Check sheet for the modelled part. Datum: model origin and axes. Units: mm. Face numbers are marked on the shaded views. A direction names the side the tool comes from. Round coordinates to 2 decimals unless told otherwise and drop trailing zeros. Order: outer loops, then holes, each group sorted by start corner. A loop starts at its lowest first (then second) coordinate and runs counter-clockwise, first axis right, second up.
```python
from build123d import *

# Parameters (mm, degrees)
F1_DEPTH = 7
F2_R     = 2.5
F3_DEPTH = 5.001
F4_R     = 0.99999


# Not quite as in the source:
# - a fillet or chamfer is up to 0.001 mm smaller than in the source, because OpenCascade refuses the exact size


with BuildPart() as f1:
    # F0 (on Right) → F1 (new body)
    with BuildSketch(Plane.YZ):
        Polygon((35, 0), (0, 0), (0, -5), (16, -5), (16, -4.25), (24.5, -4.25), (24.5, -5), (35, -5), align=None)
    extrude(amount=-F1_DEPTH)

    # F2 (on face) → F3 (cut, through all)
    with BuildSketch(Plane.XY):
        with Locations((-3.5, 7.5868815184)):
            Circle(F2_R)
    extrude(amount=-F3_DEPTH, mode=Mode.SUBTRACT)

    # F4 (radius 1 in the source; OpenCascade refuses exactly that, so slightly less here)
    f4_edges = [f1.edges().sort_by_distance(p)[0] for p in [
        (-3.5, 35, 0),
        (-7, 17.5, 0),
        (-3.5, 0, 0),
        (0, 17.5, 0),
        (0, 0, -2.5),
        (0, 35, -2.5),
        (-7, 35, -2.5),
        (-7, 0, -2.5),
    ]]
    fillet(f4_edges, radius=F4_R)


solid = f1.part
```
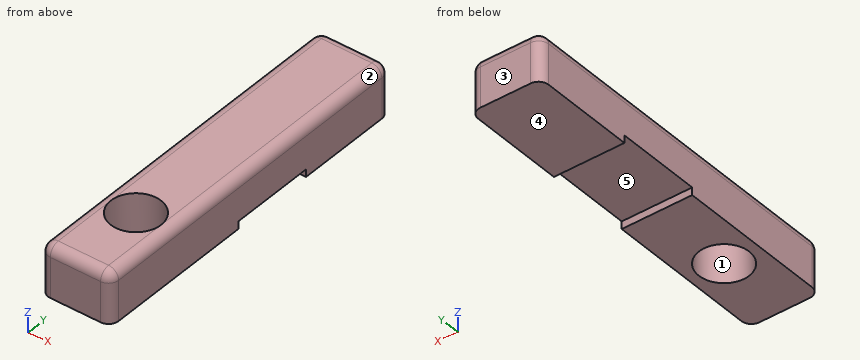
Item 1: Sectioned sample at C-C (x = -5). Record the cut outline in (y, z), and give its area (3 significant figures).
Answer:
outline: (0, -5) - (5.59, -5) - (5.59, 0) - (1, 0) arc R1 ccw to (0, -1) - close; (9.59, -5) - (16, -5) - (16, -4.25) - (24.5, -4.25) - (24.5, -5) - (35, -5) - (35, -1) arc R1 ccw to (34, 0) - (9.59, 0) - close
area: 148 mm2
Item 2: Sectioned sample at A-A (x = -3.5). Record the cut outline in (y, z), and give its area (3 significant figures).
Answer:
outline: (0, -5) - (5.09, -5) - (5.09, 0) - (1, 0) arc R1 ccw to (0, -1) - close; (10.09, -5) - (16, -5) - (16, -4.25) - (24.5, -4.25) - (24.5, -5) - (35, -5) - (35, -1) arc R1 ccw to (34, 0) - (10.09, 0) - close
area: 143 mm2
Item 3: Release check for a two-part mould opening along X. For the marked faces 1, 2 and 3 record: released by +X, released by -X, zero draft, split by the parting line, or undercut.
Answer:
face 1: undercut
face 2: released by +X
face 3: zero draft
Item 4: Scan lines: line 1 along Y through (x, z) = (-3.5, -3.15); line 2 along X through (y, z) = (6, -2.15); line 3 along Y through (x, z) = (-5.5, -0.6). Record each from-to range of solid material in increasing order.
Answer:
line 1: y = 0 to 5.09, 10.09 to 35
line 2: x = -7 to -5.43, -1.57 to 0
line 3: y = 0.08 to 6.09, 9.09 to 34.92
Item 5: Access from +Z, -Z, +X, -X, +Y, -Y to the whole of each face (thin tool, end or side, straight path). Record for the marked faces 4 and 5.
Answer:
face 4: -Z, +X, -X, +Y, -Y
face 5: -Z, +X, -X
Item 6: Sectioned sample at B-B (z = -3.45). Record the cut outline in (x, y).
Answer:
outline: (-7, 1) arc R1 ccw to (-6, 0) - (-1, 0) arc R1 ccw to (0, 1) - (0, 34) arc R1 ccw to (-1, 35) - (-6, 35) arc R1 ccw to (-7, 34) - close; hole circle Ø5 at (-3.5, 7.59)
Item 7: Sectioned sample at D-D (z = -0.5). Record the cut outline in (x, y), and give its area (3 significant figures).
Answer:
outline: (-6.87, 1) arc R0.87 ccw to (-6, 0.13) - (-1, 0.13) arc R0.87 ccw to (-0.13, 1) - (-0.13, 34) arc R0.87 ccw to (-1, 34.87) - (-6, 34.87) arc R0.87 ccw to (-6.87, 34) - close; hole circle Ø5 at (-3.5, 7.59)
area: 214 mm2
